Design review of the part built by this model. Coordinates are the model's own, in mm. A direction names the side the tool comes from. Coordinates: 2 decimals unless noted, no trailing zeros. Loops run counter-clockwise (first coordinate to the right, second up) from the corner with the lowest first, then second, coordinate; pieces in that order, holes last. Notation, with made-up numbers: (38, 88) - (78, 88) arc R20 cw to (78, 96) - close; hole circle Ø8 at (8.25, 5.25). An arc over 180 degrees is marked (long way). Answer in a Markdown table with one row per item. Add a question column.
(1) Clearance check with flat-ended pins moving along their axes: pin 1 (1 mm diameter, centred on x = 42, y = 2, fed in from +Z); pin 2 (1 mm diameter, centred on x = 52.5, y = 2.5, fed in from +Z); pin 3 (1.6 mm diameter, centred on x = 52, y = 2, fed in from +Z). State where each tip first meets the part, or that it passes through.
(2) We need section C-C, the plane y = 1.45. Give the number of separate pieces and of enclosed holes in the cut face, plus the area to 3 significant figures.
(3) To check wall thickness, follow L1, parallel to X at y = 1.2, z = -86.25; L2, parallel to Z at x = -18.5, y = 1.1; L3, parallel to Z at x = -30, y = 2.5. State the ranges of each line that lie inside material, in increasing order. Write a range as [from, to].
(4) The part is to be moulded in two halves that separate along X. For faces 1 (the face through (6.784, 1.565, -9.115)), 2 (the face through (78.83, 1.61, -108.99)), 3 (the face through (-0.396, 1.565, 25.397)), 4 (the face through (-50.93, 1.57, -45.91)), say which applies: released by +X, released by -X, zero draft, split by the parting line, or undercut.
(5) For faces 5 (the face through (21.457, 1.565, -65.281)), 6 (the face through (-1.1, 0, -49.6)), 7 (the face through (40.965, 1.565, -104.884)), list the 3-axis set-ups (+Z, -Z, +X, -X, +Y, -Y) from which the entire face can be reached by the end or side of a thin tool; tool diameter is ignored.
(6) We need section A-A, the plane x = 17.5. Write out the cut boundary in (y, z) (1 decimal), plus the area to 3 significant figures.
(7) We need section B-B, the plane z = -98.5. Write out the cut boundary in (x, y) (3 decimals), plus the area to 3 significant figures.
(8) We need section D-D, the plane x = -25. Write out the cut boundary in (y, z) (3 decimals).
from build123d import *

# Parameters (mm, degrees)
SKETCH1_R               = 1.65
SKETCH1_R_2             = 1.6
SKETCH1_W               = 9
SKETCH1_H               = 9
SKETCH1_R_3             = 3
SKETCH1_R_4             = 7.6
SKETCH1_R_5             = 2.6
BOSS_EXTRUDE1_DEPTH     = 3.175
FILLET1_R               = 10
CUT_EXTRUDE1_DEPTH      = 1
CUT_EXTRUDE1_DEPTH_BACK = 4.175


with BuildPart() as part:
    # Sketch1 → Boss-Extrude1 (new body)
    with BuildSketch(Plane(origin=(0, 0, 0), x_dir=(1, 0, 0), z_dir=(0, 1, 0))):
        with BuildLine():
            Line((-51.31658538, 125.897213638), (-82.713802404, 110.430644428))
            Line((-82.713802404, 110.430644428), (-22.785408926, -11.224310227))
            ThreePointArc((-22.785408926, -11.224310227), (0, -25.4), (22.785408926, -11.224310227))
            Line((22.785408926, -11.224310227), (82.713802404, 110.430644428))
            Line((82.713802404, 110.430644428), (51.31658538, 125.897213638))
            Line((51.31658538, 125.897213638), (34.864798721, 92.5))
            Line((34.864798721, 92.5), (-34.864798721, 92.5))
            Line((-34.864798721, 92.5), (-51.31658538, 125.897213638))
        make_face()
        Polygon((-28.707179242, 80), (28.707179242, 80), (14, 50.144348614), (-14, 50.144348614), align=None, mode=Mode.SUBTRACT)
        with Locations((-8, -8)):
            Circle(SKETCH1_R, mode=Mode.SUBTRACT)
        with Locations((-8, 8)):
            Circle(SKETCH1_R, mode=Mode.SUBTRACT)
        with Locations((-3.1, 20.76053754)):
            Circle(SKETCH1_R_2, mode=Mode.SUBTRACT)
        with Locations((8, -8)):
            Circle(SKETCH1_R, mode=Mode.SUBTRACT)
        Rectangle(SKETCH1_W, SKETCH1_H, mode=Mode.SUBTRACT)
        with Locations((8, 8)):
            Circle(SKETCH1_R, mode=Mode.SUBTRACT)
        with Locations((17.5, 29.51053754)):
            Circle(SKETCH1_R_3, mode=Mode.SUBTRACT)
        with Locations((-30, 66.453060464)):
            Circle(SKETCH1_R, mode=Mode.SUBTRACT)
        with Locations((-60, 103.923048454)):
            Circle(SKETCH1_R_4, mode=Mode.SUBTRACT)
        with Locations((30, 66.453060464)):
            Circle(SKETCH1_R, mode=Mode.SUBTRACT)
        with Locations((60, 103.923048454)):
            Circle(SKETCH1_R_4, mode=Mode.SUBTRACT)
        with Locations((0, 86.25)):
            Circle(SKETCH1_R_5, mode=Mode.SUBTRACT)
        with Locations((-3.1, 38.26053754)):
            Circle(SKETCH1_R_2, mode=Mode.SUBTRACT)
    extrude(amount=BOSS_EXTRUDE1_DEPTH)

    # Fillet1
    fillet1_edges = [part.edges().sort_by_distance(p)[0] for p in [
        (51.31658538, 1.5875, -125.897213638),
        (82.713802404, 1.5875, -110.430644428),
        (-82.713802404, 1.5875, -110.430644428),
        (-51.31658538, 1.5875, -125.897213638),
    ]]
    fillet(fillet1_edges, radius=FILLET1_R)

    # Sketch2 → Cut-Extrude1 (cut, two sides)
    with BuildSketch(Plane(origin=(0, 3.175, 0), x_dir=(1, 0, 0), z_dir=(0, 1, 0))) as cut_extrude1_sk:
        Polygon((-46.79480762, 60.144348614), (-30.073580398, 60.144348614), (-12.254779912, 23.972089701), (-20.615393523, 7), align=None)
        Polygon((-62.733510758, 92.5), (-48.694138346, 64), (-40.333524735, 80.972089701), (-46.012283536, 92.5), align=None)
        Polygon((30.073580398, 60.144348614), (46.79480762, 60.144348614), (35.218483, 36.644348614), (26.857869389, 53.616438315), align=None)
        Polygon((46.012283536, 92.5), (62.733510758, 92.5), (48.694138346, 64), (40.333524735, 80.972089701), align=None)
    extrude(amount=CUT_EXTRUDE1_DEPTH, mode=Mode.SUBTRACT)
    extrude(cut_extrude1_sk.sketch, amount=-CUT_EXTRUDE1_DEPTH_BACK, mode=Mode.SUBTRACT)


solid = part.part
Responses:
| question | item | result |
|---|---|---|
| 1 | pin 1 | stops at z = -26.77 |
| 1 | pin 2 | stops at z = -48.08 |
| 1 | pin 3 | stops at z = -46.46 |
| 2 | separate pieces | 1 |
| 2 | enclosed holes | 18 |
| 2 | area | 8,900 mm2 |
| 3 | L1 | x = [-70.8, -59.65], [-42.93, -2.6], [2.6, 42.93], [59.65, 70.8] |
| 3 | L2 | z = [-92.5, -80], [-59.28, -36.65], [-11.29, 17.4] |
| 3 | L3 | z = [-92.5, -68.1], [-64.8, -59.99], [-26.05, -3.42] |
| 4 | face 1 | undercut |
| 4 | face 2 | released by +X |
| 4 | face 3 | split by the parting line |
| 4 | face 4 | released by -X |
| 5 | face 5 | +Y, -Y |
| 5 | face 6 | +Z, -Z, +X, -X, -Y |
| 5 | face 7 | -Z, +Y, -Y |
| 6 | outline | (0, -92.5) - (3.2, -92.5) - (3.2, -80) - (0, -80) - close; (0, -57.2) - (3.2, -57.2) - (3.2, -32.5) - (0, -32.5) - close; (0, -26.5) - (3.2, -26.5) - (3.2, 18.4) - (0, 18.4) - close |
| 6 | area | 261 mm2 |
| 7 | outline | (-76.837, 0) - (-65.325, 0) - (-65.325, 3.175) - (-76.837, 3.175) - close; (-54.675, 0) - (-37.82, 0) - (-37.82, 3.175) - (-54.675, 3.175) - close; (37.82, 0) - (54.675, 0) - (54.675, 3.175) - (37.82, 3.175) - close; (65.325, 0) - (76.837, 0) - (76.837, 3.175) - (65.325, 3.175) - close |
| 7 | area | 180 mm2 |
| 8 | outline | (0, -92.5) - (3.175, -92.5) - (3.175, -80) - (0, -80) - close; (0, -72.474) - (3.175, -72.474) - (3.175, -49.845) - (0, -49.845) - close; (0, -15.901) - (3.175, -15.901) - (3.175, 6.729) - (0, 6.729) - close |
